Answer from the drawing. Dimensions are ordinates in mm from the lowest x, y and z of the part. A direction names the side the tool comes from. Round coordinates to 2 decimals unless told otherwise and drop trailing zeros. Loops run counter-clockwise (first coordinate to the right, second up) from the corner with the lowest first, then second, coordinate; pieces in that order, holes last. Notation, with made-up numbers: (31.5, 75.5) - (64.5, 75.5) arc R25 cw to (64.5, 88.5) - close; hole circle Ø2 at (76, -7.5). An arc over 180 degrees is marked (long way). Use CSV: the item, a comma, the result in double quotes. Start each with the question number.
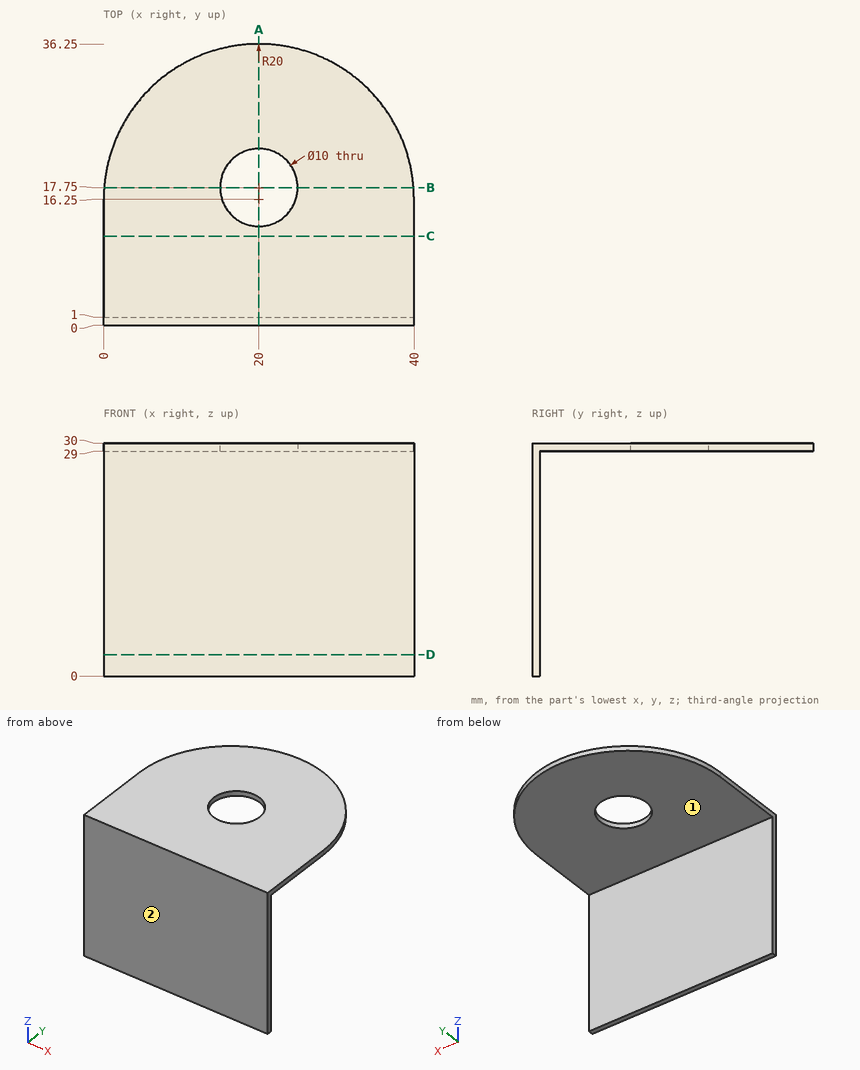
Item 1: A cutting plane is placed at B-B (y = 17.75). Determine the outline of the cut face in (x, z), plus the area to 3 significant figures.
Item 2: Each of these flat-tipped pins is pushed along its axis until it touches: pin 1 Ø10 at (x, z) = (10.5, 12.5) entering from +Y; pin 2 Ø2 at (x, y) = (25, 26.5) entering from -Z; pin 3 Ø6 at (x, y) = (20, 17.75) entering from +Z. Where does it stop, or does it pass through?
Item 3: A cutting plane is placed at C-C (y = 11.5). Determine the outline of the cut face in (x, z), plus the area to 3 significant figures.
Item 4: A cutting plane is placed at A-A (x = 20). Determine the outline of the cut face in (y, z).
Item 5: Find the intervals of material crossed by probe 1 along Y at (x, z) = (20, 29.35); probe 2 along Z at (x, y) = (11, 10.5); probe 3 along Y at (x, z) = (12.5, 27), in increasing order. Write a range as [from, to].
Item 6: A cutting plane is placed at D-D (z = 2.75). Determine the outline of the cut face in (x, y).
Item 7: Which of the six approach directions +Z, -Z, +X, -X, +Y, -Y give full straight-line access (tool end or side, diameter ignored) to the marked faces 1 and 2?
Result sheet:
1,outline,"(0.06, 29) - (15, 29) - (15, 30) - (0.06, 30) - close; (25, 29) - (39.94, 29) - (39.94, 30) - (25, 30) - close"
1,area,"29.9 mm^2"
2,pin 1,"y = 1"
2,pin 2,"z = 29"
2,pin 3,"through"
3,outline,"(0, 29) - (40, 29) - (40, 30) - (0, 30) - close"
3,area,"40.0 mm^2"
4,outline,"(0, 0) - (1, 0) - (1, 29) - (12.75, 29) - (12.75, 30) - (0, 30) - close; (22.75, 29) - (36.25, 29) - (36.25, 30) - (22.75, 30) - close"
5,probe 1,"[0, 12.75], [22.75, 36.25]"
5,probe 2,"[29, 30]"
5,probe 3,"[0, 1]"
6,outline,"(0, 0) - (40, 0) - (40, 1) - (0, 1) - close"
7,face 1,"-Z, +X, -X, +Y"
7,face 2,"+Z, -Z, +X, -X, -Y"
